Check sheet for the modelled part. Datum: model origin and axes. Units: mm. A direction names the side the tool comes from. Coordinates: 2 decimals unless noted, no trailing zeros. Loops run counter-clockwise (first coordinate to the right, second up) from the corner with the lowest first, then second, coordinate; pieces in that order, holes last. Notation, with made-up numbers: (-4, -11) - (4, -11) arc R13 ccw to (4, -1) - close; hole circle Ø4 at (48, 44). An arc over 180 degrees is marked (long way). Write each question's results on one line, items separated by ' | '. Start each with the question number.
1. Tool access check on faces 4 (the face through (-2.71, 11.32, 2.96)), 5 (the face through (0, 9.5, 9)), 6 (the face through (2.872, 6.479, 8.132)). Record the directions out of +Z, -Z, +X, -X, +Y, -Y that give a thin tool (end or side, any length) a straight path to the whole face; none if there is none.
2. Cross-section at A-A (y = 12.5). Record the cut outline in (x, z).
3. Draft check along Y on faces 1 (the face through (2.71, 13.68, 2.96)), 2 (the face through (0, 15.5, 3)), 3 (the face through (0, 7, 12)). Enter one of: released by +Y, released by -Y, zero draft, split by the parting line, or undercut.
4. Thickness scan on line 1 (X direction, y = 11.25, z = 5.25); line 2 (X direction, y = 5.7, z = 5); line 3 (Y direction, x = 4, z = 1.4). Record the ranges inside material, lowest first. Write a range as [from, to].
5. Cross-section at C-C (x = -3.25). Record the cut outline in (y, z).
6. Cross-section at D-D (x = 7.5). Record the cut outline in (y, z).
7. Cross-section at B-B (z = 5). Record the cut outline in (x, y), and give its area (3 significant figures).
8. Gauge pin test, flat end, axial feed: P1, Ø3, axis at x = 4, y = 12.5, coming from the -Z side. Record the tip position at first contact, or that the pin passes through.
```python
from build123d import *

# Parameters (mm, degrees)
SKETCH1_W           = 20
SKETCH1_H           = 10.5
SKETCH1_R           = 1.75
BOSS_EXTRUDE1_DEPTH = 12
CUT_EXTRUDE1_START  = -6
SKETCH2_W           = 20
SKETCH2_H           = 6
SKETCH2_R           = 1.75
CUT_EXTRUDE1_DEPTH  = 6
SKETCH3_R           = 4.25
CUT_EXTRUDE3_DEPTH  = 3


with BuildPart() as part:
    # Sketch1 → Boss-Extrude1 (new body)
    with BuildSketch(Plane.XY):
        with Locations((0, 10.25)):
            Rectangle(SKETCH1_W, SKETCH1_H)
        with Locations((4, 12.5)):
            Circle(SKETCH1_R, mode=Mode.SUBTRACT)
        with Locations(Location((-4, 12.5, 0), (0, 0, 180))):
            Circle(SKETCH1_R, mode=Mode.SUBTRACT)
    extrude(amount=BOSS_EXTRUDE1_DEPTH)

    # Sketch2 → Cut-Extrude1 (cut)
    with BuildSketch(Plane.XY.offset(12).offset(CUT_EXTRUDE1_START)):
        with Locations((0, 12.5)):
            Rectangle(SKETCH2_W, SKETCH2_H)
        with Locations(Location((-4, 12.5, 0), (0, 0, 180))):
            Circle(SKETCH2_R, mode=Mode.SUBTRACT)
        with Locations((4, 12.5)):
            Circle(SKETCH2_R, mode=Mode.SUBTRACT)
    extrude(amount=CUT_EXTRUDE1_DEPTH, mode=Mode.SUBTRACT)

    # Sketch3 → Cut-Extrude3 (cut)
    with BuildSketch(Plane.XZ.offset(-5)):
        with Locations(Location((0, 5, 0), (0, 0, 270))):
            Circle(SKETCH3_R)
    extrude(amount=-CUT_EXTRUDE3_DEPTH, mode=Mode.SUBTRACT)


solid = part.part
```
Established:
1) face 4: +Z, -Z | face 5: +Z, +X, -X, +Y | face 6: -Y
2) outline: (-10, 0) - (-5.75, 0) - (-5.75, 6) - (-10, 6) - close; (-2.25, 0) - (2.25, 0) - (2.25, 6) - (-2.25, 6) - close; (5.75, 0) - (10, 0) - (10, 6) - (5.75, 6) - close
3) face 1: undercut | face 2: released by +Y | face 3: zero draft
4) line 1: [-10, -5.22], [-2.78, 2.78], [5.22, 10] | line 2: [-10, -4.25], [4.25, 10] | line 3: [5, 10.75], [14.25, 15.5]
5) outline: (5, 0) - (10.92, 0) - (10.92, 6) - (9.5, 6) - (9.5, 12) - (5, 12) - (5, 7.74) - (8, 7.74) - (8, 2.26) - (5, 2.26) - close; (14.08, 0) - (15.5, 0) - (15.5, 6) - (14.08, 6) - close
6) outline: (5, 0) - (15.5, 0) - (15.5, 6) - (9.5, 6) - (9.5, 12) - (5, 12) - close
7) outline: (-10, 5) - (-4.25, 5) - (-4.25, 8) - (4.25, 8) - (4.25, 5) - (10, 5) - (10, 15.5) - (-10, 15.5) - close; hole circle Ø3.5 at (-4, 12.5); hole circle Ø3.5 at (4, 12.5) | area: 165 mm^2
8) P1: through
